from build123d import *

# Parameters (mm, degrees)
F0_W           = 124.1753287613
F0_H           = 90.0488961488
F1_DEPTH       = 150
F2_R           = 25
F4_D           = 15.5
F4_CSINK_D     = 30.8
F4_CSINK_ANGLE = 90
F6_SIZE        = 25


with BuildPart() as f1:
    # F0 (on Front) → F1 (new body)
    with BuildSketch(Plane.XZ):
        with Locations((0.5159582943, 17.5197338685)):
            Rectangle(F0_W, F0_H)
    extrude(amount=F1_DEPTH)

    # F2
    f2_edges = [f1.edges().sort_by_distance(p)[0] for p in [
        (0.515958, -150, 62.544182),
        (62.603623, -75, 62.544182),
        (-61.571706, -75, 62.544182),
    ]]
    fillet(f2_edges, radius=F2_R)

    # F4 (through all)
    with Locations(Plane.XY.offset(62.5441819429)):
        with Locations((0, -84.8435163498)):
            CounterSinkHole(F4_D / 2, F4_CSINK_D / 2, counter_sink_angle=F4_CSINK_ANGLE)

    # F5: F1 across plane


with BuildPart() as f1_1:
    add(f1.part)
    add(f1.part.mirror(Plane.XZ))

    # F6
    f6_edges = [f1_1.edges().sort_by_distance(p)[0] for p in [
        (62.603623, 0, -27.504714),
        (0.515958, 150, -27.504714),
        (0.515958, -150, -27.504714),
        (-61.571706, 0, -27.504714),
    ]]
    chamfer(f6_edges, length=F6_SIZE)


solid = f1_1.part
Build history of the part. All positions in model axes, mm. Coordinates: 2 decimals unless noted, no trailing zeros. Order: outer loops, then holes, each group sorted by start corner. A loop starts at its lowest first (then second) coordinate and runs counter-clockwise, first axis right, second up. Notation, with made-up numbers: M -9,33.5 L -3,33.5 A13 ccw -3,54.5 Z; hole C 32.25,53.25 d3. An arc over 180 degrees is marked long. One line per question, with ' | ' between items. Start each with the question number.
Q1. Saw through at D-D (x = 53). List the corners of the cut face in (y, z).
Q2. Saw through at C-C (z = -15). List the corners of the cut face in (x, y).
Q3. Two-plate mould, pull along Y, no slides. Class faces 1 (the face through (-0.353, 137.325, -15.18)), 2 (the face through (1.4, -142.5, 55.4)), 3 (the face through (1.8, 92.8, 55.3)), 4 (the face through (0, -2, -27.505)): +Y half, -Y half, draft (parallel to the pull), parting line (faces both ways), or undercut.
Q4. Saw through at B-B (y = -35). List the corners of the cut face in (x, z), then the cut area to 3 significant figures.
Q5. Flat gauge pins, fed straight in: pin 1 Ø5 at (x, z) = (38, 47.5) entering from -Y; pin 2 Ø25 at (x, y) = (0, -84.84) entering from +Z; pin 3 Ø1 at (x, y) = (40, 106.5) entering from -Z. Where does each tip first touch, or does it go through?
Q6. Probe L1, parallel to Y at x = 0, z = -2.5; L2, parallel to X at y = 89.5, z = -13; L3, parallel to Z at x = 46.5, y = -129. List the from-to ranges inside material, lowest first. Write a range as from..to.
Q7. Saw through at A-A (x = 0). List the corners of the cut face in (y, z).
Check values:
1) outline: M -150,-2.5 L -140.4,-12.11 L 140.4,-12.11 L 150,-2.5 L 150,37.54 A25 ccw 140.4,57.24 L -140.4,57.24 A25 ccw -150,37.54 Z
2) outline: M -49.08,-137.5 L 50.11,-137.5 L 50.11,137.5 L -49.08,137.5 Z; hole C 0,-84.84 d15.5; hole C 0,84.84 d15.5
3) face 1: +Y half | face 2: -Y half | face 3: undercut | face 4: draft
4) outline: M -61.57,-2.5 L -36.57,-27.5 L 37.6,-27.5 L 62.6,-2.5 L 62.6,37.54 A25 ccw 37.6,62.54 L -36.57,62.54 A25 ccw -61.57,37.54 Z | area: 10,300 mm2
5) pin 1: stops at y = -148.86 | pin 2: stops at z = 59.65 | pin 3: stops at z = -25.61
6) L1: y = -150..-92.59, -77.09..77.09, 92.59..150 | L2: x = -51.08..-6.2, 6.2..52.11 | L3: z = -18.61..60.91
7) outline: M -150,-2.5 L -125,-27.5 L -92.59,-27.5 L -92.59,54.89 L -100.24,62.54 L -125,62.54 A25 ccw -150,37.54 Z; M -77.09,-27.5 L 77.09,-27.5 L 77.09,54.89 L 69.44,62.54 L -69.44,62.54 L -77.09,54.89 Z; M 92.59,-27.5 L 125,-27.5 L 150,-2.5 L 150,37.54 A25 ccw 125,62.54 L 100.24,62.54 L 92.59,54.89 Z
